```python
from build123d import *

# Parameters (mm, degrees)
SKETCH4_W = 6
SKETCH4_H = 1.5


with BuildPart() as part:
    # Sweep1: sweep along a path in Sketch1
    with BuildLine(Plane.XY) as sweep1_path:
        Line((328.167855181, -316.381930234), (-30.687774041, -316.381930234))
        ThreePointArc((-30.687774041, -316.381930234), (-35.195579771, -318.249124504), (-37.062774041, -322.756930234))
        Line((-37.062774041, -322.756930234), (-37.062774041, -703.985411885))
        ThreePointArc((-37.062774041, -703.985411885), (-35.195579771, -708.493217615), (-30.687774041, -710.360411885))
        Line((-30.687774041, -710.360411885), (431.312225959, -710.360411885))
        ThreePointArc((431.312225959, -710.360411885), (435.820031689, -708.493217615), (437.687225959, -703.985411885))
        Line((437.687225959, -703.985411885), (437.687225959, -148.660411885))
        ThreePointArc((437.687225959, -148.660411885), (435.820031689, -144.152606155), (431.312225959, -142.285411885))
        Line((431.312225959, -142.285411885), (377.312225959, -142.285411885))
        ThreePointArc((377.312225959, -142.285411885), (372.112225959, -147.485411885), (377.312225959, -152.685411885))
        Line((377.312225959, -152.685411885), (414.812225959, -152.685411885))
        ThreePointArc((414.812225959, -152.685411885), (419.479130714, -154.618507129), (421.412225959, -159.285411885))
        Line((421.412225959, -159.285411885), (421.412225959, -309.931930234))
        ThreePointArc((421.412225959, -309.931930234), (419.479130714, -314.59883499), (414.812225959, -316.531930234))
        Line((414.812225959, -316.531930234), (362.867855181, -316.531930234))
    # Sketch4 → Sweep1 (sweep)
    with BuildSketch(Plane(origin=(328.167855181, -316.381930234, 0), x_dir=(0, 0, -1), z_dir=(1, 0, 0))):
        Rectangle(SKETCH4_W, SKETCH4_H)
    sweep(path=sweep1_path.line)


solid = part.part
```
Geometry: final body of the model. Coordinates: model frame, mm. Coordinates: 2 decimals unless noted, no trailing zeros. Write each loop counter-clockwise with the first axis right and the second up, starting at its lowest first coordinate (ties: lowest second). Pieces come first, ordered by that corner, then holes. Notation, with made-up numbers: M 42,63 L 50,63 A23 cw 50,80 Z; hole C -18.75,8.5 d2. An arc over 180 degrees is marked long. Use CSV: the item, a comma, the result in double quotes. Start each with the question number.
1. First-contact query: P1, Ø1.2, axis at y = -316.5, z = -1.5, coming from the -X side; P2, Ø1.8, axis at x = 109.5, z = 0.5, coming from the +Y side. Flat tips, straight axial feed; report the tip coordinate or a pass-through.
2. Cut plane D-D on x = 129. Return the cut outline in (y, z), plus the area to 3 significant figures.
3. Cut plane B-B on x = 402.5. Return the cut outline in (y, z).
4. Cut plane A-A on y = -378. Return the cut outline in (x, z).
5. Ray query, probe 1 along Y at (x, z) = (387, 1); probe 2 along Y at (x, z) = (64.5, 1.6); probe 3 along X at (y, z) = (-495.5, -1.1). Return the intervals inside material, ascending.
Entries:
1,P1,"x = -35.02"
1,P2,"y = -315.63"
2,outline,"M -711.11,-3 L -709.61,-3 L -709.61,3 L -711.11,3 Z; M -317.13,-3 L -315.63,-3 L -315.63,3 L -317.13,3 Z"
2,area,"18.0 mm²"
3,outline,"M -711.11,-3 L -709.61,-3 L -709.61,3 L -711.11,3 Z; M -317.28,-3 L -315.78,-3 L -315.78,3 L -317.28,3 Z; M -153.44,-3 L -151.94,-3 L -151.94,3 L -153.44,3 Z; M -143.04,-3 L -141.54,-3 L -141.54,3 L -143.04,3 Z"
4,outline,"M -37.81,-3 L -36.31,-3 L -36.31,3 L -37.81,3 Z; M 436.94,-3 L 438.44,-3 L 438.44,3 L 436.94,3 Z"
5,probe 1,"-711.11 to -709.61, -317.28 to -315.78, -153.44 to -151.94, -143.04 to -141.54"
5,probe 2,"-711.11 to -709.61, -317.13 to -315.63"
5,probe 3,"-37.81 to -36.31, 436.94 to 438.44"
